from build123d import *

# Parameters (mm, degrees)
SKETCH1_R           = 4
BOSS_EXTRUDE1_DEPTH = 170
SKETCH2_R           = 5
BOSS_EXTRUDE2_DEPTH = 5
BOSS_EXTRUDE3_START = -18
SKETCH3_R           = 4
BOSS_EXTRUDE3_DEPTH = 18


with BuildPart() as part:
    # Sketch1 → Boss-Extrude1 (new body)
    with BuildSketch(Plane.XY):
        Circle(SKETCH1_R)
    extrude(amount=BOSS_EXTRUDE1_DEPTH)

    # Sketch2 → Boss-Extrude2 (add)
    with BuildSketch(Plane.XY):
        Circle(SKETCH2_R)
    extrude(amount=-BOSS_EXTRUDE2_DEPTH)

    # Sketch3 → Boss-Extrude3 (add)
    with BuildSketch(Plane.XY.offset(BOSS_EXTRUDE3_START)):
        Circle(SKETCH3_R)
    extrude(amount=BOSS_EXTRUDE3_DEPTH)


solid = part.part
Check sheet for the modelled part. Datum: model origin and axes. Units: mm. A direction names the side the tool comes from. Give positions to 0.01 mm unless a question says otherwise; leave off trailing zeros. Order: outer loops, then holes, each group sorted by start corner. A loop starts at its lowest first (then second) coordinate and runs counter-clockwise, first axis right, second up. Notation, with made-up numbers: (4, 45) - (19, 45) arc R22 cw to (19, 65) - close; hole circle Ø1 at (-27, 66). An arc over 180 degrees is marked (long way). Answer as CSV lines item,"result".
1. Go/stop test with flat-tipped pins: P1, Ø1.5, axis at y = -1, z = 137.5, coming from the -X side; P2, Ø6, axis at x = 0.5, z = 130.5, coming from the +Y side; P3, Ø2, axis at x = 3.5, y = 2.5, coming from the -Z side. Record where each tip stops, or that it passes through.
Result sheet:
P1,"x = -3.99"
P2,"y = 4"
P3,"z = -18"
2. Section check C-C (z = 37). Record the boundary of the cut face in (x, y), then the cut area to 3 significant figures.
Result sheet:
outline,"circle Ø8 at (0, 0)"
area,"50.3 mm²"
3. Section check A-A (y = 0). Record the boundary of the cut face in (x, z), then the cut area to 3 significant figures.
Result sheet:
outline,"(-5, -5) - (-4, -5) - (-4, -18) - (4, -18) - (4, -5) - (5, -5) - (5, 0) - (4, 0) - (4, 170) - (-4, 170) - (-4, 0) - (-5, 0) - close"
area,"1,510 mm²"
4. Scan lines: probe 1 along Z at (x, y) = (3.25, 3.5); probe 2 along Y at (x, z) = (0.5, 25.5). Record each from-to range of solid material in increasing order. Write a range as from..to.
Result sheet:
probe 1,"-5..0"
probe 2,"-3.97..3.97"
5. Tool access check on faces 1 (the face through (-0.867, -3.905, 83.81)), 2 (the face through (0, 0, 170)), 3 (the face through (-0.867, -3.905, -11.591)). Record the directions out of +Z, -Z, +X, -X, +Y, -Y that give a thin tool (end or side, any length) a straight path to the whole face; none if there is none.
Result sheet:
face 1,"+Z"
face 2,"+Z, +X, -X, +Y, -Y"
face 3,"-Z"
